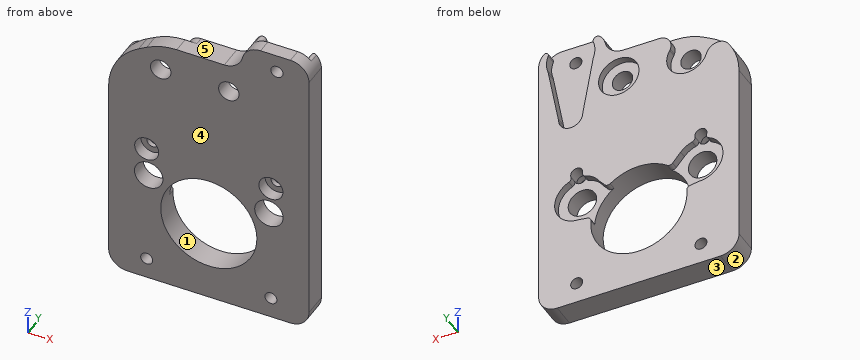
from build123d import *

# Parameters (mm, degrees)
SKETCH1_R           = 3.55
SKETCH1_R_2         = 12
SKETCH1_R_3         = 1.5
SKETCH1_R_4         = 2.55
BOSS_EXTRUDE1_DEPTH = 6
SKETCH2_R           = 5.05
CUT_EXTRUDE1_DEPTH  = 1.8
SKETCH11_R          = 1.52
CUT_EXTRUDE9_DEPTH  = 13
SKETCH14_W          = 37.681595327
SKETCH14_H          = 11.476856365
CUT_EXTRUDE13_DEPTH = 10
FILLET1_R           = 4.635
FILLET2_R           = 4.635
SKETCH15_R          = 3
CUT_EXTRUDE14_DEPTH = 3
CHAMFER1_SIZE       = 7.5
CHAMFER1_SIZE2      = 12.990381057
FILLET4_R           = 15
CUT_EXTRUDE15_START = 6
CUT_EXTRUDE15_DEPTH = 2
FILLET5_R           = 3
FILLET6_R           = 1
CUT_EXTRUDE16_START = 6
CUT_EXTRUDE16_DEPTH = 2.5
FILLET7_R           = 1
FILLET8_R           = 0.7
FILLET9_R           = 10


with BuildPart() as part:
    # Sketch1 → Boss-Extrude1 (new body)
    with BuildSketch(Plane(origin=(0, 0, 0), x_dir=(1, 0, 0), z_dir=(0, 1, 0))):
        with BuildLine():
            Line((-20.365, 45), (20.365, 45))
            ThreePointArc((20.365, 45), (23.642439931, 43.642439931), (25, 40.365))
            Line((25, 40.365), (25, -24.635))
            ThreePointArc((25, -24.635), (23.642439931, -27.912439931), (20.365, -29.27))
            Line((20.365, -29.27), (-20.365, -29.27))
            Line((-20.365, -29.27), (-25, -29.27))
            Line((-25, -29.27), (-25, -20.365))
            Line((-25, -20.365), (-25, 40.365))
            ThreePointArc((-25, 40.365), (-23.642439931, 43.642439931), (-20.365, 45))
        make_face()
        with Locations(Location((-15, 15.95, 0), (0, 0, 270))):
            Circle(SKETCH1_R, mode=Mode.SUBTRACT)
        with Locations(Location((0, 24.25, 0), (0, 0, 270))):
            Circle(SKETCH1_R_2, mode=Mode.SUBTRACT)
        with Locations(Location((15.5, 39.75, 0), (0, 0, 270))):
            Circle(SKETCH1_R_3, mode=Mode.SUBTRACT)
        with Locations(Location((-15.5, 39.75, 0), (0, 0, 90))):
            Circle(SKETCH1_R_3, mode=Mode.SUBTRACT)
        with Locations(Location((15.5, 8.75, 0), (0, 0, 90))):
            Circle(SKETCH1_R_3, mode=Mode.SUBTRACT)
        with Locations(Location((-15.5, 8.75, 0), (0, 0, 270))):
            Circle(SKETCH1_R_3, mode=Mode.SUBTRACT)
        with Locations(Location((5, -14.95, 0), (0, 0, 270))):
            Circle(SKETCH1_R_4, mode=Mode.SUBTRACT)
        with Locations(Location((15, 15.95, 0), (0, 0, 90))):
            Circle(SKETCH1_R, mode=Mode.SUBTRACT)
        with Locations(Location((-12, -14.95, 0), (0, 0, 90))):
            Circle(SKETCH1_R_4, mode=Mode.SUBTRACT)
    extrude(amount=BOSS_EXTRUDE1_DEPTH)

    # Sketch2 → Cut-Extrude1 (cut)
    with BuildSketch(Plane(origin=(0, 6, 0), x_dir=(1, 0, 0), z_dir=(0, 1, 0))):
        with Locations(Location((5, -14.95, 0), (0, 0, 270))):
            Circle(SKETCH2_R)
        with Locations(Location((-12, -14.95, 0), (0, 0, 270))):
            Circle(SKETCH2_R)
        with BuildLine():
            Line((-7.5, 23.1), (-15, 21.95))
            ThreePointArc((-15, 21.95), (-20.935673069, 16.826233541), (-16.733678611, 10.205928406))
            Line((-16.733678611, 10.205928406), (-16.932966202, 9.193404855))
            Line((-16.932966202, 9.193404855), (-14, 8.75))
            Line((-14, 8.75), (-14.130110059, 10.013393942))
            ThreePointArc((-14.130110059, 10.013393942), (-12.101208946, 10.696714321), (-10.441369548, 12.048860628))
            Line((-10.441369548, 12.048860628), (-5.220684774, 18.149430314))
            Line((-5.220684774, 18.149430314), (-7.5, 23.1))
        make_face()
        with BuildLine():
            Line((4.956760879, 18.508794553), (9.839172222, 12.889631289))
            ThreePointArc((9.839172222, 12.889631289), (11.659255417, 10.966083304), (14.130110059, 10.013393942))
            Line((14.130110059, 10.013393942), (14, 8.75))
            Line((14, 8.75), (16.988984535, 8.931452623))
            Line((16.988984535, 8.931452623), (16.718687374, 10.201425071))
            ThreePointArc((16.718687374, 10.201425071), (20.936810995, 16.818490192), (15, 21.95))
            Line((15, 21.95), (7.5, 23.1))
            Line((7.5, 23.1), (4.956760879, 18.508794553))
        make_face()
    extrude(amount=-CUT_EXTRUDE1_DEPTH, mode=Mode.SUBTRACT)

    # Sketch11 → Cut-Extrude9 (cut)
    with BuildSketch(Plane(origin=(0, 0, 0), x_dir=(1, 0, 0), z_dir=(0, 1, 0))):
        with Locations(Location((17, -24.772297108, 0), (0, 0, 270))):
            Circle(SKETCH11_R)
    extrude(amount=CUT_EXTRUDE9_DEPTH, mode=Mode.SUBTRACT)

    # Sketch14 → Cut-Extrude13 (cut)
    with BuildSketch(Plane(origin=(0, 0, 0), x_dir=(1, 0, 0), z_dir=(0, 1, 0))):
        with Locations((-10.340797664, -27.738428183)):
            Rectangle(SKETCH14_W, SKETCH14_H)
    extrude(amount=CUT_EXTRUDE13_DEPTH, mode=Mode.SUBTRACT)

    # Fillet1
    fillet1_edges = [part.edges().sort_by_distance(p)[0] for p in [
        (8.5, 3, 22),
    ]]
    fillet(fillet1_edges, radius=FILLET1_R)

    # Fillet2
    fillet2_edges = [part.edges().sort_by_distance(p)[0] for p in [
        (8.5, 3, 29.27),
    ]]
    fillet(fillet2_edges, radius=FILLET2_R)

    # Sketch15 → Cut-Extrude14 (cut)
    with BuildSketch(Plane(origin=(0, 0, 0), x_dir=(1, 0, 0), z_dir=(0, 1, 0))):
        with Locations(Location((-15.5, 8.75, 0), (0, 0, 270))):
            Circle(SKETCH15_R)
        with Locations(Location((15.5, 8.75, 0), (0, 0, 270))):
            Circle(SKETCH15_R)
    extrude(amount=CUT_EXTRUDE14_DEPTH, mode=Mode.SUBTRACT)

    # Chamfer1
    chamfer1_edges = [part.edges().sort_by_distance(p)[0] for p in [
        (-25, 3, 22),
    ]]
    chamfer1_side = [part.faces().sort_by_distance(p)[0] for p in [
        (-25, 3, -9.1825),
    ]]
    chamfer(chamfer1_edges, length=CHAMFER1_SIZE, length2=CHAMFER1_SIZE2, reference=chamfer1_side[0])

    # Fillet4
    fillet4_edges = [part.edges().sort_by_distance(p)[0] for p in [
        (-12.009618943, 3, 22),
        (-25, 3, 14.5),
    ]]
    fillet(fillet4_edges, radius=FILLET4_R)

    # Sketch16 → Cut-Extrude15 (cut)
    with BuildSketch(Plane(origin=(0, 0, 0), x_dir=(1, 0, 0), z_dir=(0, 1, 0)).offset(CUT_EXTRUDE15_START)):
        with BuildLine():
            Line((-16.664609357, -13.015078929), (-20.669862741, -22.670740182))
            Line((-20.669862741, -22.670740182), (-11.293848706, -27.720919461))
            Line((-11.293848706, -27.720919461), (-7.723076168, -17.635222996))
            ThreePointArc((-7.723076168, -17.635222996), (-9.681809366, -10.463521182), (-16.664609357, -13.015078929))
        make_face()
    extrude(amount=-CUT_EXTRUDE15_DEPTH, mode=Mode.SUBTRACT)

    # Fillet5
    # the kernel refuses this fillet: 3 mm, written as the material it takes off along each edge
    with BuildSketch(Plane(origin=(-9.249648628, 16.565462004, 21.947048042), x_dir=(0.3337437483266481, 0, -0.9426638374589739), z_dir=(0, -1, 0))) as fillet5_piece_1:
        with BuildLine():
            CenterArc((4.188427656, 3), FILLET5_R, 160.503835971, 109.496164029)
            Line((1.360436144, 4.001231245), (1.077636993, 4.101354369))
            ThreePointArc((1.077636993, 4.101354369), (0.087557633, 1.30486151), (-0.290206287, 0.076028357))
            Line((-0.290206287, 0.076028357), (0, -0.3))
            Line((0, -0.3), (4.188427656, -0.3))
            Line((4.188427656, -0.3), (4.188427656, 0))
        make_face()
    extrude(amount=12.565462004, mode=Mode.SUBTRACT)
    with BuildSketch(Plane(origin=(-18.743864962, 18.470022706, 18.027642644), x_dir=(0.3831526873327851, 0, -0.9236850210919656), z_dir=(0, -1, 0))) as fillet5_piece_2:
        with BuildLine():
            CenterArc((4.461410952, -3), FILLET5_R, 90, 122.26907024)
            ThreePointArc((1.92476045, -4.601687931), (0.769762504, -2.381410701), (0, 0))
            Line((0, 0), (4.461410952, 0))
        make_face()
    extrude(amount=14.470022706, mode=Mode.SUBTRACT)

    # Fillet6
    fillet6_edges = [part.edges().sort_by_distance(p)[0] for p in [
        (-14.130110059, 5.1, -10.013393942),
        (-16.733678611, 5.1, -10.205928406),
        (14.130110059, 5.1, -10.013393942),
        (16.718687374, 5.1, -10.201425071),
        (11.861373055, 5.1, -22.431256132),
        (7.852565986, 5.1, -15.176014799),
        (-7.802278744, 5.1, -15.132739095),
        (-11.861373055, 5.1, -22.431256132),
    ]]
    fillet(fillet6_edges, radius=FILLET6_R)

    # Sketch17 → Cut-Extrude16 (cut)
    with BuildSketch(Plane(origin=(0, 0, 0), x_dir=(1, 0, 0), z_dir=(0, 1, 0)).offset(CUT_EXTRUDE16_START)):
        with BuildLine():
            Line((11.327335926, -22.66911326), (14, -7.772297108))
            ThreePointArc((14, -7.772297108), (17, -4.772297108), (20, -7.772297108))
            Line((20, -7.772297108), (22.672664074, -22.66911326))
            ThreePointArc((22.672664074, -22.66911326), (17, -30.822297108), (11.327335926, -22.66911326))
        make_face()
    extrude(amount=-CUT_EXTRUDE16_DEPTH, mode=Mode.SUBTRACT)

    # Fillet7
    # the kernel refuses this fillet: 1 mm, written as the material it takes off along each edge
    with BuildSketch(Plane(origin=(12.953622769, 3.5, 29.27), x_dir=(-0.9295463102395678, 0, -0.36870537983599505), z_dir=(0, 1, 0))) as fillet7_piece_1:
        with BuildLine():
            CenterArc((3.110158636, -0.926607536), FILLET7_R, 67.912019708, 154.403348054)
            Line((2.370708081, -1.599818408), (2.296763026, -1.667139495))
            ThreePointArc((2.296763026, -1.667139495), (1.225310358, -0.740699506), (-0.034759798, -0.093764367))
            Line((-0.034759798, -0.093764367), (-0.036870538, 0.092954631))
            ThreePointArc((-0.036870538, 0.092954631), (-0.002529968, 0.106575849), (3.523791509, 0.092660754))
            Line((3.523791509, 0.092660754), (3.48618852, 0))
        make_face()
    extrude(amount=11.215471301, mode=Mode.SUBTRACT)

    # Fillet8
    fillet8_edges = [part.edges().sort_by_distance(p)[0] for p in [
        (21.112884992, 4.75, 29.209264207),
    ]]
    fillet(fillet8_edges, radius=FILLET8_R)

    # Fillet9
    fillet9_edges = [part.edges().sort_by_distance(p)[0] for p in [
        (22.672664074, 4.75, 22.66911326),
        (20, 4.75, 7.772297108),
        (11.327335926, 4.75, 22.66911326),
        (14, 4.75, 7.772297108),
    ]]
    fillet(fillet9_edges, radius=FILLET9_R)


solid = part.part
Design review of the part built by this model. Coordinates are the model's own, in mm. Face numbers are marked on the shaded views. A direction names the side the tool comes from. Give positions to 0.01 mm unless a question says otherwise; leave off trailing zeros. Write each loop counter-clockwise with the first axis right and the second up, starting at its lowest first coordinate (ties: lowest second). Pieces come first, ordered by that corner, then holes. Notation, with made-up numbers: M 62.5,57 L 114.5,57 A29 ccw 114.5,88 Z; hole C 21.25,72 d10. An arc over 180 degrees is marked long. Return JSON: item names as keys, results as strings. Group by question number.
Item 1: Take a section at A-A (z = -24.25). Give the boundary of the cut face in (x, y), plus the area to 3 significant figures.
Item 2: The part is to be moulded in two halves that separate along X. For the marked faces 1, 2 and 3, say which applies: pulls with the +X half, pulls with the -X half, needs draft (parallel to the pull), parting line crosses it, or undercut.
Item 3: Take a section at B-B (x = 5). Give the boundary of the cut face in (y, z).
Item 4: Tool access review of the marked faces 4 and 5: name each direction out of +Z, -Z, +X, -X, +Y, -Y from which nothing blocks a thin tool from reaching the whole face with its end or side.
Item 5: Wall thickness on line 1 along X through (y, z) = (3.45, -39.75); line 2 along X through (y, z) = (1.5, -8.75); line 3 along X through (y, z) = (1.5, -17.5): over which ranges is each line inside the solid? List them lowest first.
Item 6: Take a section at D-D (y = 5.25). Count the separate pieces of the cut face and the enclosed holes in it, plus the area to 3 significant figures.
Item 7: Clearance check with flat-ended pins moving along their axes: pin 1 Ø4.5 at (x, z) = (5, 14.95) entering from +Y (3 decimals); pin 2 Ø6 at (x, z) = (-12, 14.95) entering from +Y; pin 3 Ø5 at (x, z) = (-15.5, -8.75) entering from -Y; pin 4 Ø3 at (x, z) = (4, 14) entering from +Y. State where each tip first meets the part, or that it passes through.
Item 8: Take a section at C-C (x = -19.5). Give the boundary of the cut face in (y, z).
Return value:
{
 "1": {"outline": "M -25,0 L -12,0 L -12,6 L -25,6 Z; M 12,0 L 25,0 L 25,6 L 12,6 Z", "area": "156 mm2"},
 "2": {"face 1": "undercut", "face 2": "pulls with the -X half", "face 3": "needs draft"},
 "3": {"outline": "M 0,-45 L 6,-45 L 6,-35.16 L 0,-35.16 Z; M 0,-13.34 L 6,-13.34 L 6,9.9 L 4.2,9.9 L 4.2,12.4 L 0,12.4 Z; M 0,17.5 L 4.2,17.5 L 4.2,20 L 6,20 L 6,22.14 L 0,22.14 Z"},
 "4": {"face 4": "+Z, -Z, +X, -X, -Y", "face 5": "+Z, -X, +Y, -Y"},
 "5": {"line 1": "x = -25 to -17, -14 to 14, 17 to 25", "line 2": "x = -25 to -18.5, -12.5 to 12.5, 18.5 to 25", "line 3": "x = -25 to -18.19, -11.81 to -9.92, 9.92 to 11.81, 18.19 to 25"},
 "6": {"separate pieces": "1", "enclosed holes": "4", "area": "2,270 mm2"},
 "7": {"pin 1": "passes through", "pin 2": "stops at y = 4", "pin 3": "stops at y = 3", "pin 4": "stops at y = 4.2"},
 "8": {"outline": "M 0,-45 L 6,-45 L 6,-19.92 L 4.2,-19.92 L 4.2,-11.98 L 6,-11.98 L 6,15.74 L 4,15.74 L 4,17.45 L 0,17.45 Z"}
}
